Autodesk Inventor part; units mm, degrees
ref_plane "YZ Plane" through (0, 0, 0) normal (1, 0, 0) x (0, 1, 0)
ref_plane "XZ Plane" through (0, 0, 0) normal (0, 1, 0) x (-1, 0, 0)
ref_plane "XY Plane" through (0, 0, 0) normal (0, 0, 1) x (1, 0, 0)
sketch "Sketch1" plane through (0, 0, 0) normal (0, 1, 0) x (-1, 0, 0)
  line L0 (0, 0) -> (17.272, 0)
  line L1 (17.272, 0) -> (17.272, -12.7)
  line L2 (17.272, -12.7) -> (0, -12.7)
  line L3 (0, -12.7) -> (0, 0)
  circle A0 centre (21.272, -10.95) radius 1.75
  circle A1 centre (-4, -1.75) radius 1.75
  line L4 (17.272, -6.35) -> (0, -6.35) construction
  circle A2 centre (21.272, -10.95) radius 2.75
  line L5 (18.272, -13.7) -> (18.272, 1)
  line L6 (18.272, 1) -> (-1, 1)
  line L7 (-1, 1) -> (-1, -13.7)
  line L8 (-1, -13.7) -> (18.272, -13.7)
  line L9 (18.272, -13.7) -> (21.272, -13.7)
  line L10 (21.272, -8.2) -> (18.272, -8.2)
  circle A3 centre (-4, -1.75) radius 2.75
  line L11 (-1, 1) -> (-4, 1)
  line L12 (-4, -4.5) -> (-1, -4.5)
  dimension "d0" = 17.272
  dimension "d1" = 12.7
  dimension "d2" = 3.5
  dimension "d3" = 3.5
  dimension "d4" = 4
  dimension "d5" = 4
  dimension "d6" = 5.5
  dimension "d7" = 5.5
extrude "Extrusion1" add sketch "Sketch1" along normal blind 2 contours L0 L1 L2 L3 | A2 | A2 L9 L5 L10 | L5 L8 L7 L6 | L7 L12 A3 L11 | A3
equation "\"d3\" = d2"
equation "\"d5\" = d4"
equation "\"d7\" = d6"
properties part number "USB Mount"
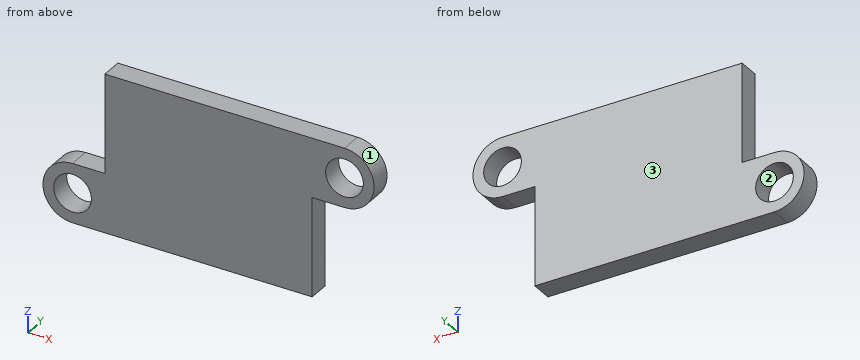
Model file for the job. Use its own axes, mm. Face numbers are marked on the shaded views. Give positions to 0.01 mm unless a question says otherwise; leave off trailing zeros. Loops run counter-clockwise (first coordinate to the right, second up) from the corner with the lowest first, then second, coordinate; pieces in that order, holes last. Notation, with made-up numbers: (1, 74.5) - (43, 74.5) arc R28 cw to (43, 96.5) - close; hole circle Ø8 at (87.25, 7.5). An arc over 180 degrees is marked (long way). One line per item, written item: value. Start each with the question number.
1. Pull direction X, two halves, no side cores. Call the marked faces 1, 2 and 3: pulls with the +X half, pulls with the -X half, needs draft (parallel to the pull), parting line crosses it, or undercut.
2. Probe L1, parallel to Z at x = 4, y = 1.55; L2, parallel to X at y = 1.8, z = -6.75; L3, parallel to Z at x = -22, y = 1.05. List the from-to ranges inside material, lowest first. Write a range as from..to.
3. Pin check, flat tips, straight feed: pin 1 (1 mm diameter, centred on y = 1, z = -10, fed in from +X); pin 2 (0.6 mm diameter, centred on x = 3, y = 1.5, fed in from -Z); pin 3 (3 mm diameter, centred on x = -21.272, z = -10.95, fed in from +Y); pin 4 (1 mm diameter, centred on x = -20, y = 0.5, fed in from +Z). Stop position of each tip, or through.
4. Slice it at B-B (y = 1.3). List the corners of the cut face in (x, z), plus the area to 3 significant figures.
5. Slice it at C-C (x = 5). List the corners of the cut face in (y, z), plus the area to 3 significant figures.
6. Slice it at A-A (z = -10.95). List the corners of the cut face in (x, y), plus the area to 3 significant figures.
7. Slice it at D-D (z = -6.75). List the corners of the cut face in (x, y).
Solution:
1. face 1: pulls with the +X half
1. face 2: undercut
1. face 3: needs draft
2. L1: z = -4.5..-3.5, 0..1
2. L2: x = -18.27..1
2. L3: z = -13.6..-12.54, -9.36..-8.3
3. pin 1: stops at x = 1
3. pin 2: stops at z = -4.5
3. pin 3: passes through
3. pin 4: stops at z = -8.2
4. outline: (-21.27, -13.7) - (1, -13.7) - (1, -4.5) - (4, -4.5) arc R2.75 ccw to (4, 1) - (-18.27, 1) - (-18.27, -8.2) - (-21.27, -8.2) arc R2.75 ccw to start; hole circle Ø3.5 at (-21.27, -10.95); hole circle Ø3.5 at (4, -1.75)
4. area: 321 mm^2
5. outline: (0, -4.31) - (2, -4.31) - (2, -3.19) - (0, -3.19) - close; (0, -0.31) - (2, -0.31) - (2, 0.81) - (0, 0.81) - close
5. area: 4.50 mm^2
6. outline: (-24.02, 0) - (-23.02, 0) - (-23.02, 2) - (-24.02, 2) - close; (-19.52, 0) - (1, 0) - (1, 2) - (-19.52, 2) - close
6. area: 43.0 mm^2
7. outline: (-18.27, 0) - (1, 0) - (1, 2) - (-18.27, 2) - close
